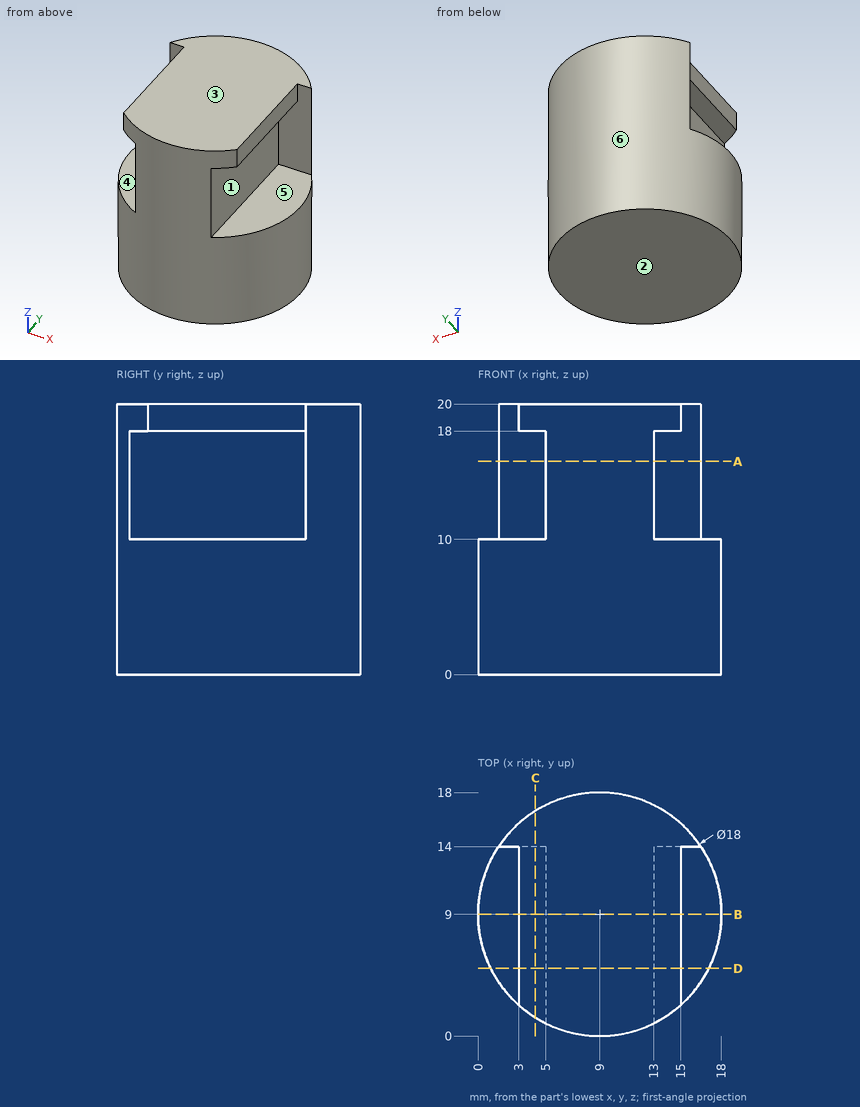
Job drawing, mm, ordinate dimensions from the low corner. One solid piece. A direction names the side the tool comes from. Give positions to 0.01 mm unless a question says otherwise; leave off trailing zeros. Write each loop counter-clockwise with the first axis right and the second up, starting at its lowest first coordinate (ties: lowest second). Pieces come first, ordered by that corner, then holes. Notation, with made-up numbers: (-21.5, 70) -> (-17.5, 70) arc R20 cw to (-17.5, 94) -> close; hole circle Ø11 at (-25, 87). An arc over 180 degrees is marked (long way). Return JSON: item names as keys, results as strings.
Item 1: Band-saw the part on B-B (y = 9). List the corners of the cut face in (x, z), then the cut area to 3 significant figures.
Answer below:
{"outline": "(0, 0) -> (18, 0) -> (18, 10) -> (13, 10) -> (13, 18) -> (15, 18) -> (15, 20) -> (3, 20) -> (3, 18) -> (5, 18) -> (5, 10) -> (0, 10) -> close", "area": "268 mm2"}
Item 2: Band-saw the part on D-D (y = 5). List the corners of the cut face in (x, z).
Answer below:
{"outline": "(0.94, 0) -> (17.06, 0) -> (17.06, 10) -> (13, 10) -> (13, 18) -> (15, 18) -> (15, 20) -> (3, 20) -> (3, 18) -> (5, 18) -> (5, 10) -> (0.94, 10) -> close"}
Item 3: Two-plate mould, pull along Z, no slides. Class the marked faces 1, 2 and 3: +Z half, -Z half, draft (parallel to the pull), parting line (faces both ways), or undercut.
Answer below:
{"face 1": "undercut", "face 2": "-Z half", "face 3": "+Z half"}
Item 4: Tool access for the marked faces 4, 5 and 6: list every direction of +Z, -Z, +X, -X, +Y, -Y with a clear straight run to the whole face (end or side of a thin tool).
Answer below:
{"face 4": "-X, -Y", "face 5": "+X, -Y", "face 6": "+Z, -Z"}
Item 5: Drill centre lines: probe 1 along Z at (x, y) = (4.25, 6.25); probe 2 along Y at (x, z) = (4, 10.5); probe 3 along X at (y, z) = (7.25, 15.5). Where is each one in solid material? Low to high.
Answer below:
{"probe 1": "z = 0 to 10, 18 to 20", "probe 2": "y = 14 to 16.48", "probe 3": "x = 5 to 13"}
Item 6: Band-saw the part on A-A (z = 15.75). List the corners of the cut face in (x, y), then the cut area to 3 significant figures.
Answer below:
{"outline": "(1.52, 14) -> (5, 14) -> (5, 0.94) arc R9 ccw to (13, 0.94) -> (13, 14) -> (16.48, 14) arc R9 ccw to start", "area": "152 mm2"}
Item 7: Band-saw the part on C-C (x = 4.25). List the corners of the cut face in (y, z).
Answer below:
{"outline": "(1.36, 0) -> (16.64, 0) -> (16.64, 20) -> (1.36, 20) -> (1.36, 18) -> (14, 18) -> (14, 10) -> (1.36, 10) -> close"}
Item 8: Drop flat-ended pins along their axis: pin 1 (6 mm diameter, centred on x = 2, z = 3, fed in from +Y); pin 2 (2 mm diameter, centred on y = 10.5, z = 19, fed in from -X); pin 3 (2.5 mm diameter, centred on y = 4.5, z = 16, fed in from -X); pin 4 (5.5 mm diameter, centred on x = 2.5, y = 10.5, fed in from +Z). Give the stop position or say it passes through.
Answer below:
{"pin 1": "stops at y = 17.06", "pin 2": "stops at x = 3", "pin 3": "stops at x = 5", "pin 4": "stops at z = 20"}
